Autodesk Inventor part; units mm, degrees
ref_plane "YZ Plane" through (0, 0, 0) normal (1, 0, 0) x (0, 1, 0)
ref_plane "XZ Plane" through (0, 0, 0) normal (0, 1, 0) x (-1, 0, 0)
ref_plane "XY Plane" through (0, 0, 0) normal (0, 0, 1) x (1, 0, 0)
sketch "Sketch1" plane through (0, 0, 0) normal (0, 0, 1) x (1, 0, 0)
  line L0 (0, 0) -> (37.0648, 0)
  line L1 (37.0648, 0) -> (37.0648, 13)
  line L2 (0, 0) -> (0, 13)
  line L3 (0, 13) -> (6.35, 13)
  line L4 (37.0648, 13) -> (30.7148, 13)
  line L5 (18.5324, 0) -> (18.5324, 24.6661)
  line L6 (6.35, 13) -> (30.7148, 13) construction
  arc A0 (6.35, 13) -> (30.7148, 13) centre (18.5324, 13) ccw
  dimension "d0" = 37.0648
  dimension "d1" = 13
  dimension "d2" = 13
  dimension "d3" = 6.35
  dimension "d4" = 6.35
  dimension "d5" = 12.1824
  dimension "d6" = 13
extrude "Extrusion1" add sketch "Sketch1" along normal blind 30.365
sketch "Sketch2" plane through (0, 0, 30.365) normal (0, 0, 1) x (1, 0, 0)
  line L0 (0, 13) -> (0, 0)
  line L1 (0, 0) -> (37.0648, 0)
  line L2 (0, 0) -> (37.0648, 0)
  line L3 (37.0648, 0) -> (37.0648, 13)
  line L4 (0, 0) -> (0, 13)
  line L5 (0, 13) -> (6.042, 13)
  arc A0 (6.35, 13) -> (30.7148, 13) centre (18.5324, 13) ccw
  line L6 (6.35, 13) -> (30.7148, 13) construction
  line L7 (18.5324, 0) -> (18.5324, 13)
  line L8 (37.0648, 13) -> (31.0228, 13)
  arc A1 (6.042, 13) -> (31.0228, 13) centre (18.5324, 13) ccw
  point P0 (0, 13)
  point P1 (37.0648, 13)
  dimension "d9" = 13
  dimension "d10" = 13
  dimension "d11" = 6.042
  dimension "d13" = 37.0648
  dimension "d15" = 6.042
  dimension "d16" = 12.4904
extrude "Extrusion2" add sketch "Sketch2" along normal blind 21.635
sketch "Sketch3" plane through (0, 0, 52) normal (0, 0, 1) x (1, 0, 0)
  line L0 (0, 0) -> (37.0648, 0)
  line L1 (0, 0) -> (37.0648, 0)
  line L2 (37.0648, 0) -> (37.0648, 32.7)
  line L3 (37.0648, 32.7) -> (0, 32.7)
  line L4 (0, 32.7) -> (0, 0)
  line L5 (18.5324, 32.7) -> (18.5324, 0)
  line L6 (0, 0) -> (37.0648, 0)
  circle A0 centre (18.5324, 21.89) radius 1.8
  circle A1 centre (18.5324, 13) radius 3.625
  circle A2 centre (18.5324, 4.491) radius 1.8
  dimension "d19" = 37.0648
  dimension "d20" = 32.7
  dimension "d21" = 7.25
  dimension "d22" = 3.6
  dimension "d23" = 3.6
  dimension "d24" = 13
  dimension "d25" = 8.509
  dimension "d26" = 8.89
extrude "Extrusion3" add sketch "Sketch3" along normal blind 2.5 contours L4 L3 L5 A0 A1 A2 L0 | L5 A2 A1 A0 L3 L2 L0
sketch "Sketch4" plane through (0, 0, 0) normal (0, -1, 0) x (1, 0, 0)
  circle A0 centre (31.9848, 48.15) radius 2
  circle A1 centre (5.08, 48.15) radius 2
  circle A2 centre (31.9848, 6.35) radius 2
  circle A3 centre (5.08, 6.35) radius 2
  line L0 (0, 54.5) -> (37.0648, 54.5)
  line L1 (37.0648, 0) -> (37.0648, 54.5)
  line L2 (0, 0) -> (37.0648, 0)
  line L3 (0, 0) -> (0, 54.5)
  dimension "d29" = 4
  dimension "d30" = 4
  dimension "d32" = 4
  dimension "d33" = 4
  dimension "d34" = 6.35
  dimension "d35" = 5.08
  dimension "d36" = 5.08
  dimension "d37" = 6.35
  dimension "d38" = 6.35
  dimension "d39" = 5.08
  dimension "d40" = 6.35
  dimension "d41" = 5.08
  dimension "d42" = 26.9048
  dimension "d43" = 41.8
extrude "Extrusion4" cut sketch "Sketch4" against normal blind 7 contours A0 | A1 | A2 | A3
equation "\"d1\" = motor_centerline_height"
equation "\"d2\" = d1"
equation "\"d24\" = motor_centerline_height"
equation "\"m3_heat_set_insert\" = 4"
equation "\"m3_clearance\" = 3.4"
equation "\"m3_heat_set_depth\" = 7"
equation "\"robot_diameter\" = 354"
equation "\"hardboard_thickness\" = 5"
equation "\"motor_centerline_height\" = 13"
properties part number "motor_holder"
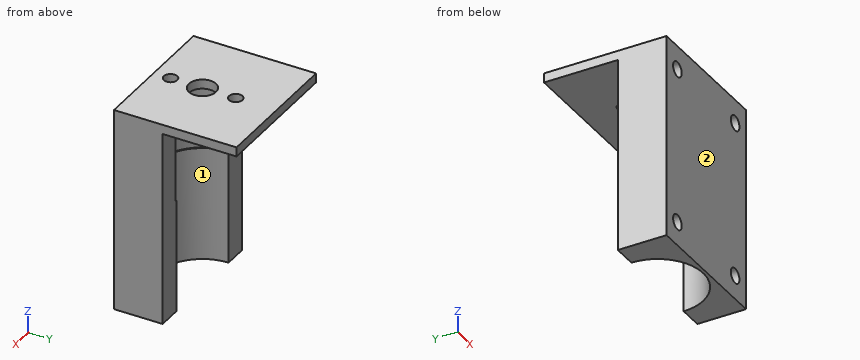
Input: part model. Units: mm. Frame: model coordinates. Face numbers are marked on the shaded views. A direction names the side the tool comes from. Give positions to 0.01 mm unless a question says otherwise; leave off trailing zeros. Write each loop counter-clockwise with the first axis right and the second up, starting at its lowest first coordinate (ties: lowest second). Pieces come first, ordered by that corner, then holes.
Q1. First-contact query: P1, Ø4, axis at x = 30, z = 28.5, coming from the +Y side; P2, Ø3.5, axis at x = 31.98, z = 48.15, coming from the -Y side; P3, Ø2, axis at x = 16.5, y = 25.5, coming from the -Z side. Flat tips, straight axial feed; report the tip coordinate or a pass-through.
Q2. Set-up query: the marked faces 1 and 2. Return all of +Z, -Z, +X, -X, +Y, -Y with unobstructed straight access to the full face (end or side cutting, diameter ignored); none if empty.
Q3. Material intervals for probe 1 along X at (y, z) = (21.89, 53); probe 2 along X at (y, z) = (5, 47.5); probe 3 along X at (y, z) = (13, 53.7), sorted ascending.
Q4. Section A-A, the plane y = 21.89. Output: boundary loops of the cut face in (x, z).
Q5. Section D-D, the plane y = 29. Output: boundary loops of the cut face in (x, z), plus the area to 3 significant figures.
Q6. Section B-B, the plane z = 21.5. Output: boundary loops of the cut face in (x, y).
Q7. Section C-C, the plane x = 5.08. Output: boundary loops of the cut face in (y, z).
Filled in:
1. P1: stops at y = 13
1. P2: stops at y = 7
1. P3: stops at z = 52
2. face 1: -Z, +Y
2. face 2: +Z, -Z, +X, -X, -Y
3. probe 1: x = 0 to 16.73, 20.33 to 37.06
3. probe 2: x = 0 to 3.19, 6.97 to 8.94, 28.12 to 30.09, 33.88 to 37.06
3. probe 3: x = 0 to 14.91, 22.16 to 37.06
4. outline: (0, 52) - (16.73, 52) - (16.73, 54.5) - (0, 54.5) - close; (20.33, 52) - (37.06, 52) - (37.06, 54.5) - (20.33, 54.5) - close
5. outline: (0, 52) - (37.06, 52) - (37.06, 54.5) - (0, 54.5) - close
5. area: 92.7 mm2
6. outline: (0, 0) - (37.06, 0) - (37.06, 13) - (30.71, 13) arc R12.18 cw to (6.35, 13) - (0, 13) - close
7. outline: (0, 0) - (13, 0) - (13, 52) - (32.7, 52) - (32.7, 54.5) - (0, 54.5) - (0, 50.15) - (7, 50.15) - (7, 46.15) - (0, 46.15) - (0, 8.35) - (7, 8.35) - (7, 4.35) - (0, 4.35) - close
